Geometry: see drawing. Coordinates: mm, zero at the bounding-box minimum. Coordinates: 2 decimals unless noted, no trailing zeros. Order: outer loops, then holes, each group sorted by start corner. A loop starts at its lowest first (then second) coordinate and runs counter-clockwise, first axis right, second up. Notation, with made-up numbers: M -14,19.25 L 13,19.25 A17 ccw 13,35.25 Z; hole C -16,5.5 d11. An arc over 180 degrees is marked long. One line per item, written item: value.
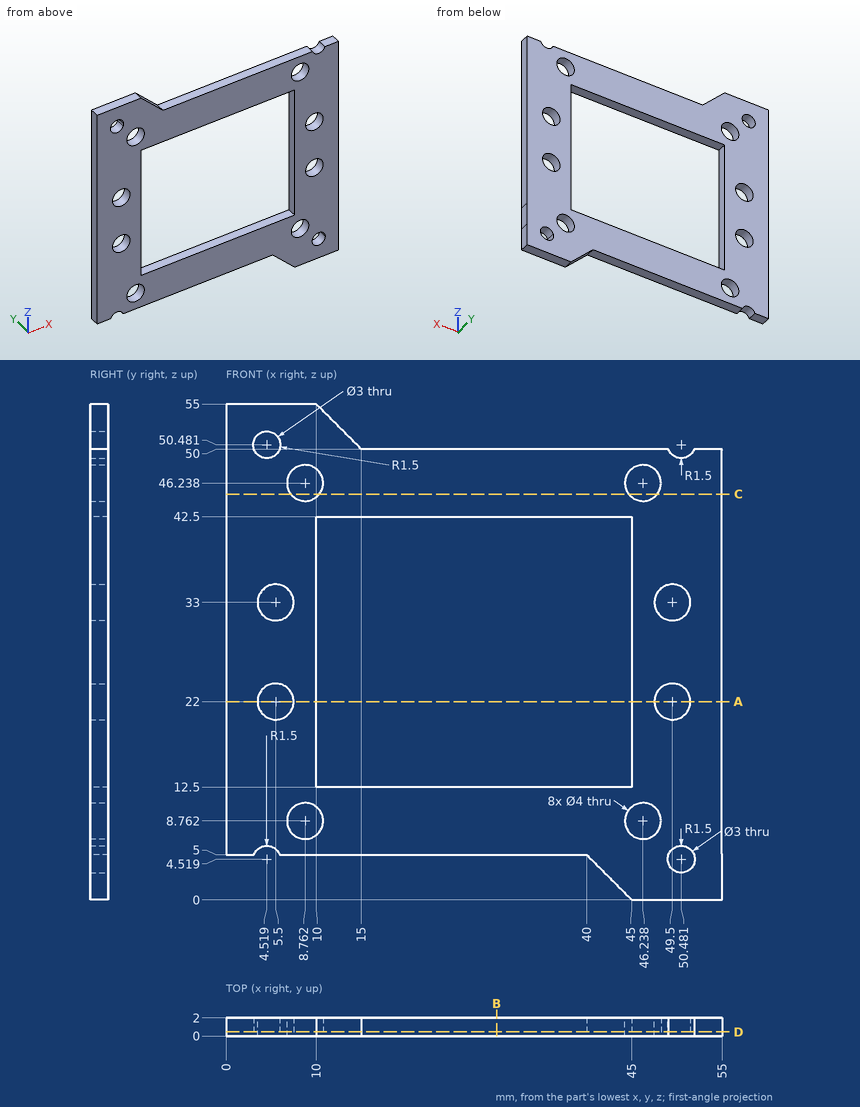
(1) First-contact query: pin 1 (5 mm diameter, centred on x = 46.24, z = 46.24, fed in from +Y); pin 2 (3 mm diameter, centred on x = 49.5, z = 33, fed in from -Y); pin 3 (1 mm diameter, centred on x = 1, y = 1.5, fed in from -Z); pin 4 (0.6 mm diameter, centred on x = 52.5, y = 1, fed in from +Z). Flat tips, straight axial feed; report the tip coordinate or a pass-through.
Data:
pin 1: stops at y = 2
pin 2: passes through
pin 3: stops at z = 5
pin 4: stops at z = 50
(2) Cut plane B-B on x = 30. Output: boundary loops of the cut face in (y, z).
Data:
outline: M 0,5 L 2,5 L 2,12.5 L 0,12.5 Z; M 0,42.5 L 2,42.5 L 2,50 L 0,50 Z
(3) Cut plane C-C on z = 45. Output: boundary loops of the cut face in (x, y).
Data:
outline: M 0,0 L 7.19,0 L 7.19,2 L 0,2 Z; M 10.33,0 L 44.67,0 L 44.67,2 L 10.33,2 Z; M 47.81,0 L 55,0 L 55,2 L 47.81,2 Z
(4) Cut plane A-A on z = 22. Output: boundary loops of the cut face in (x, y).
Data:
outline: M 0,0 L 3.5,0 L 3.5,2 L 0,2 Z; M 7.5,0 L 10,0 L 10,2 L 7.5,2 Z; M 45,0 L 47.5,0 L 47.5,2 L 45,2 Z; M 51.5,0 L 55,0 L 55,2 L 51.5,2 Z
(5) Cut plane D-D on y = 0.45. Give the number of separate pieces and of enclosed holes in the cut face, plus the area to 3 significant figures.
Data:
separate pieces: 1
enclosed holes: 11
area: 1,430 mm2
(6) Ray query, line 1 (Z direction, x = 22, y = 0.85); line 2 (X direction, y = 0.75, z = 10); line 3 (X direction, y = 1.1, z = 17). Return the intervals inside material, ascending. Write a range as from..to.
Data:
line 1: z = 5..12.5, 42.5..50
line 2: x = 0..7.19, 10.33..44.67, 47.81..55
line 3: x = 0..10, 45..55
